from build123d import *

# Parameters (mm, degrees)
F0_W     = 458.0001
F0_H     = 452.00062
F1_DEPTH = 1211.000118
F3_DEPTH = 169.999914


with BuildPart() as f1:
    # F0 (on Front) → F1 (new body)
    with BuildSketch(Plane.XZ):
        Rectangle(F0_W, F0_H)
    extrude(amount=F1_DEPTH)

    # F2 (on face) → F3 (join)
    with BuildSketch(Plane.XZ.offset(1211.000118)):
        with BuildLine():
            ThreePointArc((-10.259218514, 37.6406649164), (-23.6835473139, -31.0025935447), (39.0137311708, 0))
            ThreePointArc((39.0137311708, 0), (31.0025935447, 23.6835473139), (10.259218514, 37.6406649164))
            Line((10.259218514, 37.6406649164), (10.259218514, 30.7776723057))
            Line((10.259218514, 30.7776723057), (-10.259218514, 30.7776723057))
            Line((-10.259218514, 30.7776723057), (-10.259218514, 37.6406649164))
        make_face()
        with BuildLine():
            Line((10.259218514, 30.7776723057), (10.259218514, 37.6406649164))
            ThreePointArc((10.259218514, 37.6406649164), (0, 39.0137311708), (-10.259218514, 37.6406649164))
            Line((-10.259218514, 37.6406649164), (-10.259218514, 30.7776723057))
            Line((-10.259218514, 30.7776723057), (10.259218514, 30.7776723057))
        make_face()
        with BuildLine():
            ThreePointArc((-10.259218514, 37.6406649164), (0, 39.0137311708), (10.259218514, 37.6406649164))
            Line((10.259218514, 37.6406649164), (10.259218514, 47.2497900359))
            Line((10.259218514, 47.2497900359), (-10.259218514, 47.2497900359))
            Line((-10.259218514, 47.2497900359), (-10.259218514, 37.6406649164))
        make_face()
    extrude(amount=F3_DEPTH)


solid = f1.part
Model file for the job. Use its own axes, mm. A direction names the side the tool comes from. Round coordinates to 2 decimals unless told otherwise and drop trailing zeros. Order: outer loops, then holes, each group sorted by start corner. A loop starts at its lowest first (then second) coordinate and runs counter-clockwise, first axis right, second up. Notation, with made-up numbers: M 44,46 L 90,46 A32 cw 90,76 Z; hole C 68,84.5 d1. An arc over 180 degrees is marked long. Write each question's results on one line, items separated by ' | '. Start each with the question number.
(1) Drop flat-ended pins along their axis: pin 1 (5 mm diameter, centred on y = -1318, z = 40.5, fed in from -X); pin 2 (16.5 mm diameter, centred on x = 5, y = -1321.5, fed in from +Z); pin 3 (12 mm diameter, centred on x = 117.5, z = 116, fed in from -Y). Give the stop position or say it passes through.
(2) Saw through at B-B, the plane x = -123. Give the cut face in (y, z), then the cut area to 3 significant figures.
(3) Saw through at C-C, the plane y = -1228. Give the cut face in (x, z), then the cut area to 3 significant figures.
(4) Probe probe 1 along Y at (x, z) = (64.5, 52.5). List the from-to ranges inside material, lowest first. Write a range as from..to.
(5) Which spindle directions (+Z, -Z, +X, -X, +Y, -Y) get a long thin tool onto all of the face, cutting with end or side? Do faces 1 (the face through (-1.57, -1294.81, -38.982)), 2 (the face through (229, -597, -3)). Say none if no direction does.
(6) Saw through at A-A, the plane z = 0. Give the cut face in (x, y), then the cut area to 3 significant figures.
Established:
1) pin 1: stops at x = -10.26 | pin 2: stops at z = 47.25 | pin 3: stops at y = -1211
2) outline: M -1211,-226 L 0,-226 L 0,226 L -1211,226 Z | area: 547,000 mm^2
3) outline: M -10.26,37.64 A39.01 ccw long 10.26,37.64 L 10.26,47.25 L -10.26,47.25 Z | area: 4,960 mm^2
4) probe 1: y = -1211..0
5) face 1: -Y | face 2: +Z, -Z, +X, +Y, -Y
6) outline: M -229,-1211 L -39.01,-1211 L -39.01,-1381 L 39.01,-1381 L 39.01,-1211 L 229,-1211 L 229,0 L -229,0 Z | area: 568,000 mm^2
